Read the model definition and answer for the solid it produces. Units are mm, in the model's axes. A direction names the side the tool comes from. Coordinates: 2 decimals unless noted, no trailing zeros. Write each loop counter-clockwise with the first axis right and the second up, starting at its lowest first coordinate (ties: lowest second). Pieces come first, ordered by that corner, then holes.
Item 1: Straight lines are drawn through the part: probe 1 along Y at (x, z) = (19, 0.5); probe 2 along Z at (x, y) = (15.75, 4.35); probe 3 along X at (y, z) = (0, 3.5). For each, find the intervals that lie inside material, in ascending order.
Item 2: Section C-C (x = 15.75) is taken. Give the vertices of the cut face in (y, z), then the cut area to 3 significant figures.
Item 3: Section B-B (z = 1) is taken. Give the vertices of the cut face in (x, y), then the cut area to 3 significant figures.
Item 4: A tool of negligible diameter and unlimited length cuts with its end or side. For faces 1 (the face through (18.5, 7.27, -6.07)), 2 (the face through (10, 6, 0)), from which of +Z, -Z, +X, -X, +Y, -Y can it reach the whole face along a straight path? Write none if from no direction.
Item 5: Each of these flat-tipped pins is pushed along its axis until it touches: P1, Ø2, axis at x = -5, z = 4.5, coming from the -Y side; P2, Ø4.5, axis at x = 9.5, z = 3, coming from the -Y side; P3, Ø2, axis at x = 8, z = 1, coming from the -Y side. Where does it stop, or does it pass through?
Item 6: Section A-A (x = 12.25) is taken. Give the vertices of the cut face in (y, z).
Item 7: Section D-D (z = -4) is taken. Give the vertices of the cut face in (x, y).
Item 8: Determine the mould class of faces 3 (the face through (7.728, 3.513, -0.105)), 4 (the face through (20, 4, 0)), 5 (the face through (14, 2.5, 2)) for opening direction Y: released by +Y, released by -Y, zero draft, split by the parting line, or undercut.
from build123d import *

# Parameters (mm, degrees)
F0_R          = 6
F1_DEPTH      = 7.5
F2_SIZE       = 1
F3_SIZE       = 1
F5_DEPTH      = 49
F5_DEPTH_BACK = 15.001
F6_R          = 3
F7_W          = 20
F7_H          = 1
F8_DEPTH      = 15.001
F9_T1_DEPTH   = 53.8625025136
F10_R         = 5
F12_D         = 5


# Not quite as in the source:
# - a fillet or chamfer that OpenCascade refuses, or shapes differently, is made with other operations: its cross-section is extruded or revolved along the edge and cut away or added
# - an extrude ends at something that could not be found from the text; its depth is read off the source's solid


with BuildPart() as f1:
    # F0 (on Top) → F1 (new body, symmetric)
    with BuildSketch(Plane.XY):
        with BuildLine():
            Line((20, 8.5), (0, 8.5))
            ThreePointArc((0, 8.5), (-8.5, 0), (0, -8.5))
            Line((0, -8.5), (20, -8.5))
            Line((20, -8.5), (20, 8.5))
        make_face()
        Circle(F0_R, mode=Mode.SUBTRACT)
    extrude(amount=F1_DEPTH, both=True)

    # F2
    f2_edges = [f1.edges().sort_by_distance(p)[0] for p in [
        (-6, 0, 7.5),
    ]]
    chamfer(f2_edges, length=F2_SIZE)

    # F3
    f3_edges = [f1.edges().sort_by_distance(p)[0] for p in [
        (-6, 0, -7.5),
    ]]
    chamfer(f3_edges, length=F3_SIZE)

    # F4 (on face) → F5 (cut, two sides)
    with BuildSketch(Plane.XY.offset(7.5)) as f5_sk:
        with BuildLine():
            ThreePointArc((8.1240384046, 2.5), (6.8373971656, -5.0497524692), (0, -8.5))
            Line((0, -8.5), (20, -8.5))
            Line((20, -8.5), (20, 2.5))
            Line((20, 2.5), (8.1240384046, 2.5))
        make_face()
    extrude(amount=F5_DEPTH, mode=Mode.SUBTRACT)
    extrude(f5_sk.sketch, amount=-F5_DEPTH_BACK, mode=Mode.SUBTRACT)

    # F6
    f6_edges = [f1.edges().sort_by_distance(p)[0] for p in [
        (8.124038, 2.5, 0),
    ]]
    fillet(f6_edges, radius=F6_R)

    # F7 (on face) → F8 (cut, through all)
    with BuildSketch(Plane.XY.offset(7.5)):
        with Locations((10, 5.5)):
            Rectangle(F7_W, F7_H)
    extrude(amount=-F8_DEPTH, mode=Mode.SUBTRACT)

    # F9: fillet of radius 5.5 on 1 edges, made by hand

    # F9_s2 → F9_t1 (cut)
    with BuildSketch(Plane.XY.offset(-26.9312512568)):
        with BuildLine():
            ThreePointArc((11.4891252931, 5), (7.6855228816, 3.4727331518), (5.9943262399, -0.2608695652))
            ThreePointArc((5.9943262399, -0.2608695652), (5.3472085631, 2.7216466675), (3.3166247904, 5))
            Line((3.3166247904, 5), (11.4891252931, 5))
        make_face()
    extrude(amount=F9_T1_DEPTH, mode=Mode.SUBTRACT)

    # F10
    f10_edges = [f1.edges().sort_by_distance(p)[0] for p in [
        (20, 7.25, -7.5),
        (20, 3.75, 7.5),
        (20, 7.25, 7.5),
        (20, 3.75, -7.5),
    ]]
    fillet(f10_edges, radius=F10_R)

    # F12 (through all)
    with Locations(Plane.XZ.offset(-2.5)):
        with Locations((15.75, 0)):
            Hole(F12_D / 2)


solid = f1.part
Established:
1. probe 1: y = 2.5 to 5, 6 to 8.5
1. probe 2: z = -7.44 to -2.5, 2.5 to 7.44
1. probe 3: x = -8.5 to -6, 6.01 to 8.53
2. outline: (2.5, -7.44) - (5, -7.44) - (5, -2.5) - (2.5, -2.5) - close; (2.5, 2.5) - (5, 2.5) - (5, 7.44) - (2.5, 7.44) - close; (6, -7.44) - (8.5, -7.44) - (8.5, -2.5) - (6, -2.5) - close; (6, 2.5) - (8.5, 2.5) - (8.5, 7.44) - (6, 7.44) - close
2. area: 49.4 mm2
3. outline: (0, 6) - (13.46, 6) - (13.46, 8.5) - (0, 8.5) arc R8.5 ccw (long way) to (8.49, -0.37) arc R3 cw to (11.49, 2.5) - (13.46, 2.5) - (13.46, 5) - (11.49, 5) arc R5.5 ccw to (5.99, -0.26) arc R6 cw (long way) to start; (18.04, 2.5) - (20, 2.5) - (20, 5) - (18.04, 5) - close; (18.04, 6) - (20, 6) - (20, 8.5) - (18.04, 8.5) - close
3. area: 149 mm2
4. face 1: -Z, +X, +Y, -Y
4. face 2: +Z, -Z, +X
5. P1: stops at y = -7.5
5. P2: stops at y = -4.44
5. P3: stops at y = -4.82
6. outline: (2.5, -7.5) - (5, -7.5) - (5, 7.5) - (2.5, 7.5) - close; (6, -7.5) - (8.5, -7.5) - (8.5, 7.5) - (6, 7.5) - close
7. outline: (0, 6) - (19.77, 6) - (19.77, 8.5) - (0, 8.5) arc R8.5 ccw (long way) to (8.49, -0.37) arc R3 cw to (11.49, 2.5) - (19.77, 2.5) - (19.77, 5) - (11.49, 5) arc R5.5 ccw to (5.99, -0.26) arc R6 cw (long way) to start
8. face 3: undercut
8. face 4: zero draft
8. face 5: released by -Y
